```python
from build123d import *

# Parameters (mm, degrees)
F1_DEPTH = 5


with BuildPart() as f1:
    # F0 (on Front) → F1 (new body)
    with BuildSketch(Plane.XZ):
        with BuildLine():
            Line((-5, 89.492543), (-65, 89.492543))
            Line((-65, 89.492543), (-65, -50.507457))
            Line((-65, -50.507457), (-104.999123, -50.772287))
            Line((-104.999123, -50.772287), (-101.755198, -70.507457))
            Line((-101.755198, -70.507457), (-61.755198, -70.507457))
            ThreePointArc((-61.755198, -70.507457), (-36.016138, -39.49132), (-5, -65.23038))
            ThreePointArc((-5, -65.23038), (-4.877599, -67.868918), (-5, -70.507457))
            Line((-5, -70.507457), (125, -70.507457))
            Line((125, -70.507457), (152.5, -70.507457))
            ThreePointArc((152.5, -70.507457), (157.803301, -68.310758), (160, -63.007457))
            Line((160, -63.007457), (160, -58.007457))
            ThreePointArc((160, -58.007457), (157.803301, -52.704156), (152.5, -50.507457))
            Line((152.5, -50.507457), (125, -50.507457))
            Line((125, -50.507457), (125, -2.5))
            Line((125, -2.5), (125, 0))
            Line((125, 0), (125, 49.492543))
            Line((125, 49.492543), (75, 49.492543))
            Line((75, 49.492543), (75, 59.492543))
            Line((75, 59.492543), (95, 59.492543))
            Line((95, 59.492543), (95, 74.492543))
            Line((95, 74.492543), (55, 74.492543))
            Line((55, 74.492543), (55, 49.492543))
            Line((55, 49.492543), (-5, 49.492543))
            Line((-5, 49.492543), (-5, 89.492543))
        make_face()
    extrude(amount=F1_DEPTH)


solid = f1.part
```
Design review of the part built by this model. Coordinates are the model's own, in mm. A direction names the side the tool comes from. Give positions to 0.01 mm unless a question says otherwise; leave off trailing zeros. Loops run counter-clockwise (first coordinate to the right, second up) from the corner with the lowest first, then second, coordinate; pieces in that order, holes last. Notation, with made-up numbers: M 23,74.25 L 62,74.25 A26 ccw 62,94.25 Z; hole C -38,-19 d3. An arc over 180 degrees is marked long. Return JSON: item names as keys, results as strings. Group by question number.
Item 1: Tool access review of faces 1 (the flat face through (75, -2, 74.493)), 2 (the flat face through (-65, -2, 20)), 3 (the cylindrical face through (-4.878, -2.465, -67.832)), 4 (the flat face through (100, -2, 49.493)): name each direction out of +Z, -Z, +X, -X, +Y, -Y from which nothing blocks a thin tool from reaching the whole face with its end or side.
Item 2: Mouldability with a two-part tool opening along X and no side actions: class faces 5 (the flat face through (85, -2, 59.493)), 6 (the flat face through (95, -2, 67)), 7 (the flat face through (55, -2, 62)) as released by +X, released by -X, zero draft, split by the parting line, or undercut.
Item 3: We need section A-A (z = 67). Give the boundary of the cut face in (x, y).
Item 4: We need section D-D (z = -10). Give the boundary of the cut face in (x, y).
Item 5: We need section B-B (x = 92). Give the boundary of the cut face in (y, z), and give its area (3 significant figures).
Item 6: Insertion check: pin 1 Ø3 at (y, z) = (-3, -15.5) entering from -X; pin 2 Ø2.5 at (x, y) = (98, -3) entering from +Z; pin 3 Ø2.5 at (y, z) = (-2, 76) entering from +X. Each pin has a flat end and moves straight along its axis. Give the tip position at first contact, or say it passes through.
Item 7: For probe 1 along Z at (x, y) = (88, -0.8); probe 2 along X at (y, z) = (-3.75, 57.5); probe 3 along X at (y, z) = (-4.6, 64.5), list the stretches that pass through material, from the lowest coordinate up.
Item 8: We need section C-C (y = -1.4). Give the boundary of the cut face in (x, z), and give its area (3 significant figures).
Output:
{
 "1": {"face 1": "+Z, +X, +Y, -Y", "face 2": "+Z, -X, +Y, -Y", "face 3": "+Y, -Y", "face 4": "+X, +Y, -Y"},
 "2": {"face 5": "zero draft", "face 6": "released by +X", "face 7": "undercut"},
 "3": {"outline": "M -65,-5 L -5,-5 L -5,0 L -65,0 Z; M 55,-5 L 95,-5 L 95,0 L 55,0 Z"},
 "4": {"outline": "M -65,-5 L 125,-5 L 125,0 L -65,0 Z"},
 "5": {"outline": "M -5,-70.51 L 0,-70.51 L 0,49.49 L -5,49.49 Z; M -5,59.49 L 0,59.49 L 0,74.49 L -5,74.49 Z", "area": "675 mm^2"},
 "6": {"pin 1": "stops at x = -65", "pin 2": "stops at z = 49.49", "pin 3": "stops at x = -5"},
 "7": {"probe 1": "z = -70.51 to 49.49, 59.49 to 74.49", "probe 2": "x = -65 to -5, 55 to 75", "probe 3": "x = -65 to -5, 55 to 95"},
 "8": {"outline": "M -105,-50.77 L -101.76,-70.51 L -61.76,-70.51 A28.5 cw -5,-65.23 A28.5 cw -5,-70.51 L 152.5,-70.51 A7.5 ccw 160,-63.01 L 160,-58.01 A7.5 ccw 152.5,-50.51 L 125,-50.51 L 125,49.49 L 75,49.49 L 75,59.49 L 95,59.49 L 95,74.49 L 55,74.49 L 55,49.49 L -5,49.49 L -5,89.49 L -65,89.49 L -65,-50.51 Z", "area": "26,000 mm^2"}
}
